Can you work these out from the model? Positions are in its coordinate system, mm. A direction names the side the tool comes from. Round coordinates to 2 decimals unless told otherwise and drop trailing zeros. Loops run counter-clockwise (first coordinate to the right, second up) from the corner with the lowest first, then second, coordinate; pieces in that order, holes last.
from build123d import *

# Parameters (mm, degrees)
F0_R     = 2
F1_DEPTH = 2


with BuildPart() as f1:
    # F0 (on Top) → F1 (new body)
    with BuildSketch(Plane.XY):
        with BuildLine():
            Line((15.6879561022, 26.1114555106), (-34.3120438978, 26.1114555106))
            Line((-34.3120438978, 26.1114555106), (-34.3120438978, 16.1114555106))
            Line((-34.3120438978, 16.1114555106), (15.6879561022, 16.1114555106))
            ThreePointArc((15.6879561022, 16.1114555106), (22.4158513012, 21.1114555106), (15.6879561022, 26.1114555106))
        make_face()
        with Locations((17.1939675076, 21.1114555106)):
            Circle(F0_R, mode=Mode.SUBTRACT)
        with BuildLine():
            Line((-13.594810762, 19.7880361229), (-14.0235288377, 19.7880361229))
            Line((-14.0235288377, 19.7880361229), (-13.5748518199, 22.1032734035))
            add(Edge.make_bspline(
                [(-13.5748518199, 22.1032734035), (-13.4846374017, 22.5647241443), (-13.4127852103, 22.8521329102)],
                knots=[0, 0, 0, 1, 1, 1], degree=2))
            add(Edge.make_bspline(
                [(-13.4127852103, 22.8521329102), (-13.6395187922, 22.3803035195), (-13.7744412407, 22.1535699376)],
                knots=[0, 0, 0, 1, 1, 1], degree=2))
            Line((-13.7744412407, 22.1535699376), (-15.1412295939, 19.7880361229))
            Line((-15.1412295939, 19.7880361229), (-15.4509923749, 19.7880361229))
            Line((-15.4509923749, 19.7880361229), (-15.9124431157, 22.1535699376))
            add(Edge.make_bspline(
                [(-15.9124431157, 22.1535699376), (-15.9276119116, 22.225422129), (-16.0146328991, 22.8521329102)],
                knots=[0, 0, 0, 1, 1, 1], degree=2))
            add(Edge.make_bspline(
                [(-16.0146328991, 22.8521329102), (-16.0369869142, 22.7020416658), (-16.0892793424, 22.3838961291)],
                knots=[0, 0, 0, 1, 1, 1], degree=2))
            add(Edge.make_bspline(
                [(-16.0892793424, 22.3838961291), (-16.1415717707, 22.0657505924), (-16.5886520731, 19.7880361229)],
                knots=[0, 0, 0, 1, 1, 1], degree=2))
            Line((-16.5886520731, 19.7880361229), (-17.0125800028, 19.7880361229))
            Line((-17.0125800028, 19.7880361229), (-16.3315808992, 23.3032050011))
            Line((-16.3315808992, 23.3032050011), (-15.7423929292, 23.3032050011))
            Line((-15.7423929292, 23.3032050011), (-15.2713618962, 20.8658189949))
            add(Edge.make_bspline(
                [(-15.2713618962, 20.8658189949), (-15.2514029542, 20.7684193576), (-15.1915261279, 20.3540717201)],
                knots=[0, 0, 0, 1, 1, 1], degree=2))
            Line((-15.1915261279, 20.3540717201), (-14.932059881, 20.885777937))
            Line((-14.932059881, 20.885777937), (-13.5524978048, 23.3032050011))
            Line((-13.5524978048, 23.3032050011), (-12.9138116584, 23.3032050011))
            Line((-12.9138116584, 23.3032050011), (-13.594810762, 19.7880361229))
        make_face(mode=Mode.SUBTRACT)
        Polygon((-9.7802577527, 19.7880361229), (-10.2664575817, 19.7880361229), (-10.4540716372, 20.8163208186), (-12.0483919301, 20.8163208186), (-12.6471601923, 19.7880361229), (-13.1660926862, 19.7880361229), (-11.0504448263, 23.3032050011), (-10.5083599596, 23.3032050011), align=None, mode=Mode.SUBTRACT)
        with BuildLine():
            add(Edge.make_bspline(
                [(-6.7688525726, 20.0834284656), (-7.1879903561, 19.7377395889), (-7.8737796058, 19.7377395889)],
                knots=[0, 0, 0, 1, 1, 1], degree=2))
            add(Edge.make_bspline(
                [(-7.8737796058, 19.7377395889), (-8.454983999, 19.7377395889), (-8.7894958682, 20.0387204354)],
                knots=[0, 0, 0, 1, 1, 1], degree=2))
            add(Edge.make_bspline(
                [(-8.7894958682, 20.0387204354), (-9.1240077373, 20.3397012819), (-9.1240077373, 20.8634239219)],
                knots=[0, 0, 0, 1, 1, 1], degree=2))
            add(Edge.make_bspline(
                [(-9.1240077373, 20.8634239219), (-9.1240077373, 20.9727989245), (-9.1052463318, 21.1264827784)],
                knots=[0, 0, 0, 1, 1, 1], degree=2))
            add(Edge.make_bspline(
                [(-9.1052463318, 21.1264827784), (-9.0864849262, 21.2801666324), (-9.0665259842, 21.3719777659)],
                knots=[0, 0, 0, 1, 1, 1], degree=2))
            Line((-9.0665259842, 21.3719777659), (-8.6920962308, 23.3032050011))
            Line((-8.6920962308, 23.3032050011), (-8.2154766941, 23.3032050011))
            Line((-8.2154766941, 23.3032050011), (-8.6202440394, 21.2003308641))
            add(Edge.make_bspline(
                [(-8.6202440394, 21.2003308641), (-8.6625569966, 20.9831775743), (-8.6625569966, 20.8434649798)],
                knots=[0, 0, 0, 1, 1, 1], degree=2))
            add(Edge.make_bspline(
                [(-8.6625569966, 20.8434649798), (-8.6625569966, 20.5041629645), (-8.4442061703, 20.3145530148)],
                knots=[0, 0, 0, 1, 1, 1], degree=2))
            add(Edge.make_bspline(
                [(-8.4442061703, 20.3145530148), (-8.225855344, 20.1249430651), (-7.8338617216, 20.1249430651)],
                knots=[0, 0, 0, 1, 1, 1], degree=2))
            add(Edge.make_bspline(
                [(-7.8338617216, 20.1249430651), (-6.8758325021, 20.1249430651), (-6.6842266582, 21.1380589648)],
                knots=[0, 0, 0, 1, 1, 1], degree=2))
            Line((-6.6842266582, 21.1380589648), (-6.2650888746, 23.3032050011))
            Line((-6.2650888746, 23.3032050011), (-5.7908644109, 23.3032050011))
            Line((-5.7908644109, 23.3032050011), (-6.2147923406, 21.1101164459))
            add(Edge.make_bspline(
                [(-6.2147923406, 21.1101164459), (-6.349714789, 20.4291173423), (-6.7688525726, 20.0834284656)],
                knots=[0, 0, 0, 1, 1, 1], degree=2))
        make_face(mode=Mode.SUBTRACT)
        with BuildLine():
            Line((-4.977337932, 23.3032050011), (-3.9594318862, 23.3032050011))
            add(Edge.make_bspline(
                [(-3.9594318862, 23.3032050011), (-3.1810331453, 23.3032050011), (-2.7355495582, 22.892849152)],
                knots=[0, 0, 0, 1, 1, 1], degree=2))
            add(Edge.make_bspline(
                [(-2.7355495582, 22.892849152), (-2.2900659711, 22.482493303), (-2.2900659711, 21.7615763152)],
                knots=[0, 0, 0, 1, 1, 1], degree=2))
            add(Edge.make_bspline(
                [(-2.2900659711, 21.7615763152), (-2.2900659711, 21.1723883452), (-2.547137145, 20.7308965465)],
                knots=[0, 0, 0, 1, 1, 1], degree=2))
            add(Edge.make_bspline(
                [(-2.547137145, 20.7308965465), (-2.8042083189, 20.2894047478), (-3.2868155383, 20.0387204354)],
                knots=[0, 0, 0, 1, 1, 1], degree=2))
            add(Edge.make_bspline(
                [(-3.2868155383, 20.0387204354), (-3.7694227576, 19.7880361229), (-4.3809647428, 19.7880361229)],
                knots=[0, 0, 0, 1, 1, 1], degree=2))
            Line((-4.3809647428, 19.7880361229), (-5.6583370355, 19.7880361229))
            Line((-5.6583370355, 19.7880361229), (-4.977337932, 23.3032050011))
        make_face(mode=Mode.SUBTRACT)
    extrude(amount=F1_DEPTH)


solid = f1.part
(1) For faces 1 (the flat face through (-5.323, 21.521, 0.986)), 2 (the flat face through (-6, 20, 0)), which set-ups out of +Z, -Z, +X, -X, +Y, -Y let a thin tool reach every point of the face, with its end or its side?
Worked answers:
face 1: +Z, -Z
face 2: -Z, +X, -X, +Y, -Y
(2) If we section it at B-B, the plane y = 17: List the corners of the cut face in (x, z) for me.
Worked answers:
outline: (-34.31, 0) - (20.41, 0) - (20.41, 2) - (-34.31, 2) - close
(3) If we section it at A-A, the plane x = 5.5: List the corners of the cut face in (y, z) for me, then the cut area to 3 significant figures.
Worked answers:
outline: (16.11, 0) - (26.11, 0) - (26.11, 2) - (16.11, 2) - close
area: 20.0 mm2
(4) If we section it at C-C, the plane z = 0.4: State how many separate pieces and enclosed holes the cut face has, then the cut area to 3 significant figures.
Worked answers:
separate pieces: 1
enclosed holes: 5
area: 522 mm2
(5) Will these pins go through, and if not, where does the flat tip stop? P1, Ø0.5, axis at x = -11.5, z = 0.5, coming from the +Y side; P2, Ø0.6, axis at x = -16, z = 1, coming from the -Y side.
Worked answers:
P1: stops at y = 26.11
P2: stops at y = 16.11
(6) If we mould it in two halves opening along Y, with no side actions, what happens to faces 3 (the flat face through (-6, 20, 2)), 4 (the cylindrical face through (16.934, 23.094, 0.986)), 5 (the cylindrical face through (22.414, 20.975, 0.986))? For each: released by +Y, released by -Y, zero draft, split by the parting line, or undercut.
Worked answers:
face 3: zero draft
face 4: undercut
face 5: split by the parting line
(7) If I drill on line 1 (Y direction, x = -22, z = 0.55); line 2 (X direction, y = 19.5, z = 1.9); line 3 (X direction, y = 18, z = 1.35), over which ranges is the centre line in solid material (lowest first)?
Worked answers:
line 1: y = 16.11 to 26.11
line 2: x = -34.31 to 16.01, 18.38 to 22.16
line 3: x = -34.31 to 21.39
